```python
from build123d import *

# Parameters (mm, degrees)
F0_R     = 3
F0_R_2   = 13
F0_R_3   = 10.5
F1_DEPTH = 9
F2_R     = 3
F2_R_2   = 10.5
F3_DEPTH = 6


with BuildPart() as f1:
    # F0 (on Front) → F1 (new body)
    with BuildSketch(Plane.XZ):
        with BuildLine():
            Line((-68.315586, 54.595489), (-25.15564, -16.346062))
            ThreePointArc((-25.15564, -16.346062), (16.873102, -24.80521), (24.443739, 17.392631))
            Line((24.443739, 17.392631), (-16.17679, 84.269638))
            ThreePointArc((-16.17679, 84.269638), (-18.203137, 87.267712), (-20.575715, 90))
            Line((-20.575715, 90), (-63.424285, 90))
            ThreePointArc((-63.424285, 90), (-71.717733, 73.105646), (-68.315586, 54.595489))
        make_face()
        with Locations((-16.5, -16.5)):
            Circle(F0_R, mode=Mode.SUBTRACT)
        with Locations((16.5, -16.5)):
            Circle(F0_R, mode=Mode.SUBTRACT)
        Circle(F0_R_2, mode=Mode.SUBTRACT)
        with Locations((-16.5, 16.5)):
            Circle(F0_R, mode=Mode.SUBTRACT)
        with Locations((16.5, 16.5)):
            Circle(F0_R, mode=Mode.SUBTRACT)
        with Locations((-60, 53)):
            Circle(F0_R, mode=Mode.SUBTRACT)
        with Locations((-24, 53)):
            Circle(F0_R, mode=Mode.SUBTRACT)
        with Locations((-60, 85)):
            Circle(F0_R, mode=Mode.SUBTRACT)
        with Locations((-42, 69)):
            Circle(F0_R_3, mode=Mode.SUBTRACT)
        with Locations((-24, 85)):
            Circle(F0_R, mode=Mode.SUBTRACT)
    extrude(amount=F1_DEPTH)

    # F2 (on face) → F3 (join)
    with BuildSketch(Plane(origin=(0, 0, 0), x_dir=(-1, 0, 0), z_dir=(0, 1, 0))):
        with BuildLine():
            Line((-13.14178, 36), (57.002325, 36))
            Line((57.002325, 36), (68.315586, 54.595489))
            ThreePointArc((68.315586, 54.595489), (71.717733, 73.105646), (63.424285, 90))
            Line((63.424285, 90), (20.575715, 90))
            ThreePointArc((20.575715, 90), (18.203137, 87.267712), (16.17679, 84.269638))
            Line((16.17679, 84.269638), (-13.14178, 36))
        make_face()
        with Locations((24, 53)):
            Circle(F2_R, mode=Mode.SUBTRACT)
        with Locations((60, 53)):
            Circle(F2_R, mode=Mode.SUBTRACT)
        with Locations((42, 69)):
            Circle(F2_R_2, mode=Mode.SUBTRACT)
        with Locations((24, 85)):
            Circle(F2_R, mode=Mode.SUBTRACT)
        with Locations((60, 85)):
            Circle(F2_R, mode=Mode.SUBTRACT)
    extrude(amount=F3_DEPTH)


solid = f1.part
```
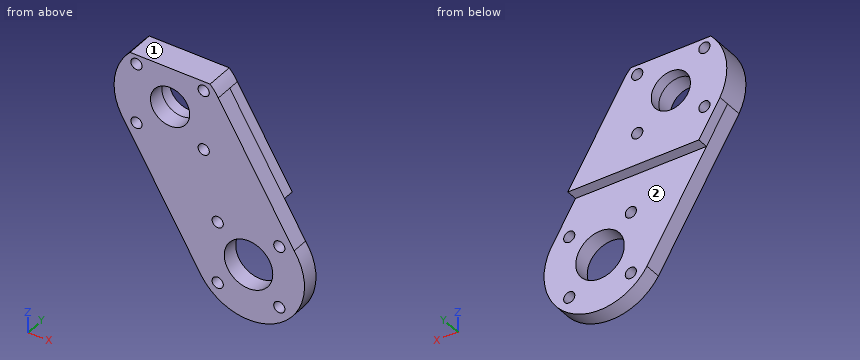
The listing builds one solid part. Answer for the finished solid, in the listing's coordinates (mm). Face numbers are marked on the shaded views. A direction names the side the tool comes from. Give positions to 0.01 mm unless a question says otherwise; leave off trailing zeros. Order: outer loops, then holes, each group sorted by start corner. A loop starts at its lowest first (then second) coordinate and runs counter-clockwise, first axis right, second up. Notation, with made-up numbers: (-18, -28.5) -> (29, -28.5) arc R27 ccw to (29, -2.5) -> close; hole circle Ø8 at (60.5, 72.25). An arc over 180 degrees is marked (long way). Answer as a JSON object with one key per item and string values. Group by question number.
Item 1: The part is cut by section C-C on y = 4.25. Write down the section's boundary in (x, z).
Item 2: A tool of negligible diameter and unlimited length cuts with its end or side. For the marked faces 1 and 2, from which of +Z, -Z, +X, -X, +Y, -Y can it reach the whole face along a straight path? Write none if from no direction.
Item 3: The part is cut by section B-B on x = 9. Write down the section's boundary in (y, z).
Item 4: Flat-ended cylindrical pins translate along their axes: pin 1 (19 mm diameter, centred on x = -42, z = 69, fed in from +Y); pin 2 (6 mm diameter, centred on y = -6, z = 62, fed in from +X); pin 3 (2 mm diameter, centred on x = -38, y = -1, fed in from -Z); pin 4 (6.5 mm diameter, centred on x = -27.5, y = 2, fed in from -Z). Find the tip coordinate at first contact, or state that the pin passes through.
Item 5: The part is cut by section D-D on x = -60. Write down the section's boundary in (y, z), and give its area (3 significant figures).
Item 6: The part is cut by section A-A on y = -6.25. Give the number of separate pieces and of enclosed holes in the cut face, and give its area (3 significant figures).
Item 7: Consider L1, parallel to Z at x = -42, y = 3.05; L2, parallel to Z at x = -16.5, y = -5.5; L3, parallel to Z at x = 17, y = -3. Determine where each line is inside the solid, lowest interval first. Write a range as from..to.
Result set:
{
 "1": {"outline": "(-68.32, 54.6) -> (-57, 36) -> (13.14, 36) -> (-16.18, 84.27) arc R30 ccw to (-20.58, 90) -> (-63.42, 90) arc R30 ccw to start; hole circle Ø6 at (-60, 53); hole circle Ø6 at (-60, 85); hole circle Ø21 at (-42, 69); hole circle Ø6 at (-24, 53); hole circle Ø6 at (-24, 85)"},
 "2": {"face 1": "+Z, +X, -X, +Y, -Y", "face 2": "-Z, +X, -X, +Y"},
 "3": {"outline": "(-9, -28.62) -> (0, -28.62) -> (0, -9.38) -> (-9, -9.38) -> close; (-9, 9.38) -> (0, 9.38) -> (0, 36) -> (6, 36) -> (6, 42.82) -> (-9, 42.82) -> close"},
 "4": {"pin 1": "through", "pin 2": "x = -0.83", "pin 3": "z = 3.12", "pin 4": "z = -16.68"},
 "5": {"outline": "(-9, 40.93) -> (6, 40.93) -> (6, 50) -> (-9, 50) -> close; (-9, 56) -> (6, 56) -> (6, 82) -> (-9, 82) -> close; (-9, 88) -> (6, 88) -> (6, 90) -> (-9, 90) -> close", "area": "556 mm²"},
 "6": {"separate pieces": "1", "enclosed holes": "10", "area": "6,300 mm²"},
 "7": {"L1": "36..58.5, 79.5..90", "L2": "-25.05..-19.5, -13.5..13.5, 19.5..84.8", "L3": "-24.72..-19.46, -13.54..13.54, 19.46..29.65"}
}
